Autodesk Inventor part; units mm, degrees
ref_plane "YZ Plane" through (0, 0, 0) normal (1, 0, 0) x (0, 1, 0)
ref_plane "XZ Plane" through (0, 0, 0) normal (0, 1, 0) x (-1, 0, 0)
ref_plane "XY Plane" through (0, 0, 0) normal (0, 0, 1) x (1, 0, 0)
sketch "Sketch1" plane through (0, 0, 0) normal (0, 0, 1) x (1, 0, 0)
  line L0 (0, 14.6647) -> (12.7, 7.3323)
  line L1 (12.7, 7.3323) -> (12.7, -7.3323)
  line L2 (12.7, -7.3323) -> (0, -14.6647)
  line L3 (0, -14.6647) -> (-12.7, -7.3323)
  line L4 (-12.7, -7.3323) -> (-12.7, 7.3323)
  line L5 (-12.7, 7.3323) -> (0, 14.6647)
  point P0 (0, 0)
  point P1 (0, 0)
  dimension "d0" = 25.4
extrude "Extrusion1" add sketch "Sketch1" along normal blind 2
sketch "Sketch2" plane through (0, 0, 2) normal (0, 0, 1) x (1, 0, 0)
  point P0 (0, 0)
hole "Hole1" at (0, 0, 2) direction (0, 0, -1) diameter 19.2532 end through all
properties part number "ETHERNET NUT"
Here's how the part is built. I have some questions about the finished solid (model axes, mm). Give positions to 0.01 mm unless a question says otherwise; leave off trailing zeros. Write each loop counter-clockwise with the first axis right and the second up, starting at its lowest first coordinate (ties: lowest second). Pieces come first, ordered by that corner, then holes. Notation, with made-up numbers: M 83.5,52.5 L 134.5,52.5 A15 cw 134.5,78.5 Z; hole C 33.5,-22 d7. An arc over 180 degrees is marked long. Put each result on its own line as item: value. Start each with the question number.
Item 1: If we section it at D-D, the plane x = -10.75: Write out the boundary of the cut face in (y, z), then the cut area to 3 significant figures.
Item 2: If we section it at B-B, the plane y = 0: Write out the boundary of the cut face in (x, z).
Item 3: If we section it at C-C, the plane x = 2: Write out the boundary of the cut face in (y, z), then the cut area to 3 significant figures.
Item 4: Will this pin go through, and if not, where does the flat tip stop? pin 1 (2 mm diameter, centred on x = 0, y = -9, fed in from -Z).
Item 5: If we section it at A-A, the plane z = 1.1: Write out the boundary of the cut face in (x, y), then the cut area to 3 significant figures.
Item 6: I need wall thicknesses on L1, parallel to X at y = 0, z = 0.7; L2, parallel to Y at x = -3.25, z = 0.4; L3, parallel to X at y = 6.5, z = 0.7. Which ranges of each line are inside material? Lowest first, please. Write a range as from..to.
Item 7: Thinking about a two-plate mould opening in X: for faces 1 (the flat face through (0, -10, 0)), 2 (the cylindrical face through (5.86, 7.64, 0.99)), 3 (the flat face through (-12.7, 0, 1)), which applies, +X half, -X half, draft (parallel to the pull), parting line (faces both ways), or undercut?
Values:
1. outline: M -8.46,0 L 8.46,0 L 8.46,2 L -8.46,2 Z
1. area: 33.8 mm²
2. outline: M -12.7,0 L -9.63,0 L -9.63,2 L -12.7,2 Z; M 9.63,0 L 12.7,0 L 12.7,2 L 9.63,2 Z
3. outline: M -13.51,0 L -9.42,0 L -9.42,2 L -13.51,2 Z; M 9.42,0 L 13.51,0 L 13.51,2 L 9.42,2 Z
3. area: 16.4 mm²
4. pin 1: z = 0
5. outline: M -12.7,-7.33 L 0,-14.66 L 12.7,-7.33 L 12.7,7.33 L 0,14.66 L -12.7,7.33 Z; hole C 0,0 d19.25
5. area: 268 mm²
6. L1: -12.7..-9.63, 9.63..12.7
6. L2: -12.79..-9.06, 9.06..12.79
6. L3: -12.7..-7.1, 7.1..12.7
7. face 1: draft
7. face 2: undercut
7. face 3: -X half
